Drawing for the job (mm, zero at the part's lowest x, y, z). A direction names the side the tool comes from. Give positions to 0.01 mm unless a question says otherwise; leave off trailing zeros. Write each loop counter-clockwise with the first axis right and the second up, starting at its lowest first coordinate (ties: lowest second). Pieces come first, ordered by that corner, then holes.
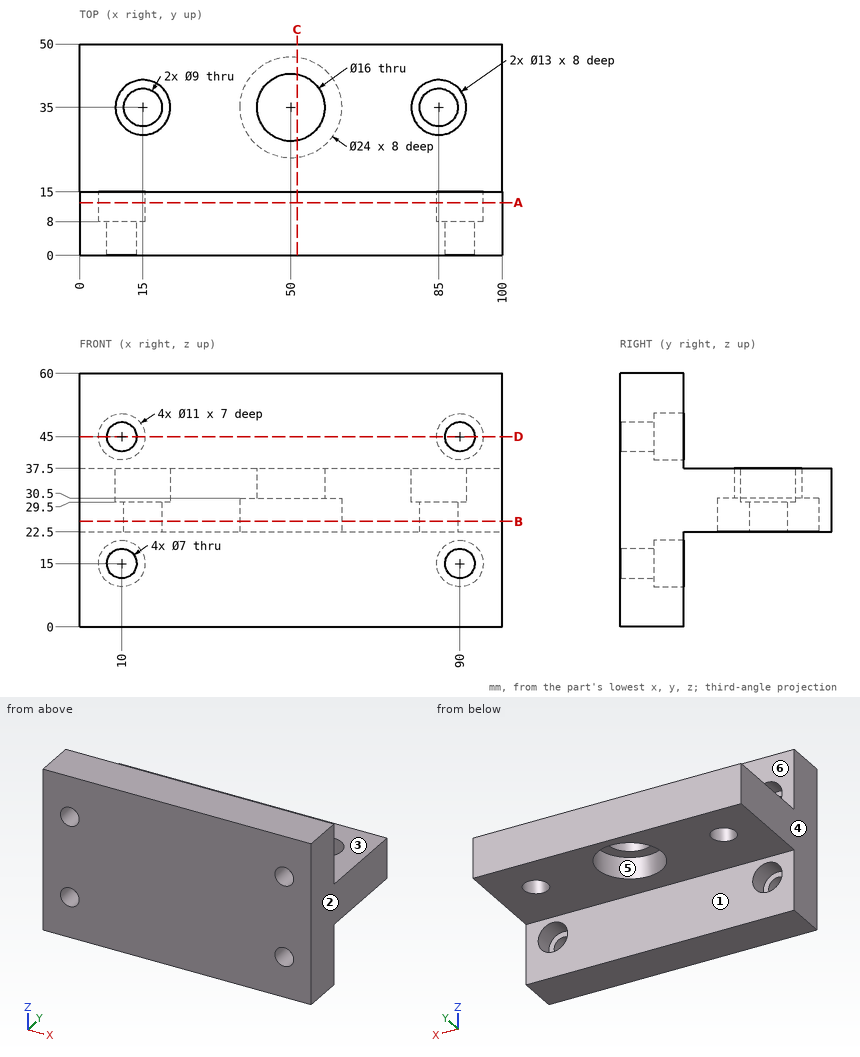
1. Pin check, flat tips, straight feed: P1, Ø17.5, axis at x = 29, y = 33, coming from the -Z side; P2, Ø3.5, axis at x = 12, z = 15, coming from the +Y side; P3, Ø19, axis at x = 50, y = 35, coming from the -Z side; P4, Ø25, axis at x = 52, z = 49, coming from the +Y side. Stop position of each tip, or through.
Calculated:
P1: stops at z = 22.5
P2: stops at y = 8
P3: stops at z = 30.5
P4: stops at y = 50
2. Slice it at A-A, the plane y = 12.5. Write the cut outline in (x, z).
Calculated:
outline: (0, 0) - (100, 0) - (100, 60) - (0, 60) - close; hole circle Ø11 at (10, 15); hole circle Ø11 at (10, 45); hole circle Ø11 at (90, 15); hole circle Ø11 at (90, 45)
3. Which spindle directions (+Z, -Z, +X, -X, +Y, -Y) get a long thin tool onto all of the face, cutting with end or side? Do the marked faces 1, 2 and 3. Say none if no direction does.
Calculated:
face 1: -Z, +X, -X, +Y
face 2: +Z, -Z, +X, +Y, -Y
face 3: +Z, +X, -X, +Y
4. Slice it at B-B, the plane z = 25. Write the cut outline in (x, y), and give its area (3 significant figures).
Calculated:
outline: (0, 0) - (100, 0) - (100, 50) - (0, 50) - close; hole circle Ø9 at (15, 35); hole circle Ø24 at (50, 35); hole circle Ø9 at (85, 35)
area: 4,420 mm2
5. Pull direction X, two halves, no side cores. Call the marked faces 4, 5 and 6: +X half, -X half, draft (parallel to the pull), parting line (faces both ways), or undercut.
Calculated:
face 4: -X half
face 5: undercut
face 6: draft
6. Slice it at D-D, the plane z = 45. Write the cut outline in (x, y), and give its area (3 significant figures).
Calculated:
outline: (0, 0) - (6.5, 0) - (6.5, 8) - (4.5, 8) - (4.5, 15) - (0, 15) - close; (13.5, 0) - (86.5, 0) - (86.5, 8) - (84.5, 8) - (84.5, 15) - (15.5, 15) - (15.5, 8) - (13.5, 8) - close; (93.5, 0) - (100, 0) - (100, 15) - (95.5, 15) - (95.5, 8) - (93.5, 8) - close
area: 1,230 mm2
7. Probe probe 1 along X at (y, z) = (5, 45); probe 2 along Z at (x, y) = (90, 48.5); probe 3 along Y at (x, z) = (68, 55). List the from-to ranges inside material, lowest first.
Calculated:
probe 1: x = 0 to 6.5, 13.5 to 86.5, 93.5 to 100
probe 2: z = 22.5 to 37.5
probe 3: y = 0 to 15
8. Slice it at C-C, the plane x = 51.5. Write the cut outline in (y, z), and give its area (3 significant figures).
Calculated:
outline: (0, 0) - (15, 0) - (15, 22.5) - (23.09, 22.5) - (23.09, 30.5) - (27.14, 30.5) - (27.14, 37.5) - (15, 37.5) - (15, 60) - (0, 60) - close; (42.86, 30.5) - (46.91, 30.5) - (46.91, 22.5) - (50, 22.5) - (50, 37.5) - (42.86, 37.5) - close
area: 1,120 mm2
